Design review of the part built by this model. Coordinates are the model's own, in mm. Face numbers are marked on the shaded views. A direction names the side the tool comes from. Coordinates: 2 decimals unless noted, no trailing zeros. Write each loop counter-clockwise with the first axis right and the second up, starting at its lowest first coordinate (ties: lowest second). Pieces come first, ordered by that corner, then holes. Notation, with made-up numbers: M 29.25,-7 L 43.25,-7 A27 cw 43.25,23 Z; hole C -27.75,33.25 d8. An arc over 180 degrees is marked long. One line per question, with ' | ' between items.
from build123d import *

# Parameters (mm, degrees)
BOSS_EXTRUDE1_DEPTH = 37
SKETCH2_R           = 2
CUT_EXTRUDE1_DEPTH  = 73.566185092
SKETCH3_W           = 30
SKETCH3_H           = 7.896551268
BOSS_EXTRUDE2_DEPTH = 48
SKETCH4_W           = 30
SKETCH4_H           = 6
CUT_EXTRUDE2_DEPTH  = 4
FILLET1_R           = 10
SKETCH5_R           = 5
CUT_EXTRUDE3_DEPTH  = 76.725712885
BOSS_EXTRUDE3_DEPTH = 1
CUT_EXTRUDE4_DEPTH  = 0.5


with BuildPart() as part:
    # Sketch1 → Boss-Extrude1 (new body)
    with BuildSketch(Plane(origin=(0, 0, 0), x_dir=(1, 0, 0), z_dir=(0, 1, 0))):
        with BuildLine():
            Line((0, 0), (6.55816832, -13.490382807))
            ThreePointArc((6.55816832, -13.490382807), (30.474828919, -7.985034321), (54.391489518, -13.490382807))
            Line((54.391489518, -13.490382807), (60.949657838, 0))
            ThreePointArc((60.949657838, 0), (30.474828919, 7.014965679), (0, 0))
        make_face()
    extrude(amount=BOSS_EXTRUDE1_DEPTH)

    # Sketch2 → Cut-Extrude1 (cut, through all)
    with BuildSketch(Plane(origin=(0, 37, 0), x_dir=(1, 0, 0), z_dir=(0, 1, 0))):
        with Locations(Location((12.985948873, -2.622359081, 0), (0, 0, 270))):
            Circle(SKETCH2_R)
        with Locations(Location((47.963708964, -2.622359081, 0), (0, 0, 90))):
            Circle(SKETCH2_R)
    extrude(amount=-CUT_EXTRUDE1_DEPTH, mode=Mode.SUBTRACT)

    # Sketch3 → Boss-Extrude2 (add)
    with BuildSketch(Plane(origin=(0, 37, 0), x_dir=(1, 0, 0), z_dir=(0, 1, 0))):
        with Locations((30.474828919, 8.066690045)):
            Rectangle(SKETCH3_W, SKETCH3_H)
    extrude(amount=-BOSS_EXTRUDE2_DEPTH)

    # Sketch4 → Cut-Extrude2 (cut)
    with BuildSketch(Plane.XY.offset(-4.118414411)):
        with Locations((30.474828919, -3)):
            Rectangle(SKETCH4_W, SKETCH4_H)
    extrude(amount=-CUT_EXTRUDE2_DEPTH, mode=Mode.SUBTRACT)

    # Fillet1
    fillet1_edges = [part.edges().sort_by_distance(p)[0] for p in [
        (15.474828919, -11, -8.066690045),
        (45.474828919, -11, -8.066690045),
    ]]
    fillet(fillet1_edges, radius=FILLET1_R)

    # Sketch5 → Cut-Extrude3 (cut, through all)
    with BuildSketch(Plane(origin=(0, 0, -12.014965679), x_dir=(-1, 0, 0), z_dir=(0, 0, -1))):
        with Locations((-30.474828919, 27)):
            Circle(SKETCH5_R)
    extrude(amount=-CUT_EXTRUDE3_DEPTH, mode=Mode.SUBTRACT)

    # Sketch7 → Boss-Extrude3 (add)
    with BuildSketch(Plane(origin=(0, 0, -12.014965679), x_dir=(-1, 0, 0), z_dir=(0, 0, -1))):
        with BuildLine():
            Line((-21.536068007, 1.453872129), (-26.199769352, 0))
            ThreePointArc((-26.199769352, 0), (-24.751375622, 3.560871216), (-21.536068007, 1.453872129))
        make_face()
        with BuildLine():
            Line((-34.426020337, 3.673663851), (-38.960174422, 5.664158065))
            ThreePointArc((-38.960174422, 5.664158065), (-37.895872331, 1.929105477), (-34.426020337, 3.673663851))
        make_face()
    extrude(amount=BOSS_EXTRUDE3_DEPTH)

    # Sketch8 → Cut-Extrude4 (cut)
    with BuildSketch(Plane(origin=(0, 0, -13.014965679), x_dir=(-1, 0, 0), z_dir=(0, 0, -1))):
        with BuildLine():
            Line((-23.022731531, 0.990416495), (-25.036897729, 0.362516061))
            ThreePointArc((-25.036897729, 0.362516061), (-24.475304572, 2.105499822), (-23.022731531, 0.990416495))
        make_face()
        with BuildLine():
            Line((-35.750767501, 4.255228023), (-37.89390211, 5.196064386))
            ThreePointArc((-37.89390211, 5.196064386), (-37.451768412, 3.29185708), (-35.750767501, 4.255228023))
        make_face()
    extrude(amount=-CUT_EXTRUDE4_DEPTH, mode=Mode.SUBTRACT)


solid = part.part
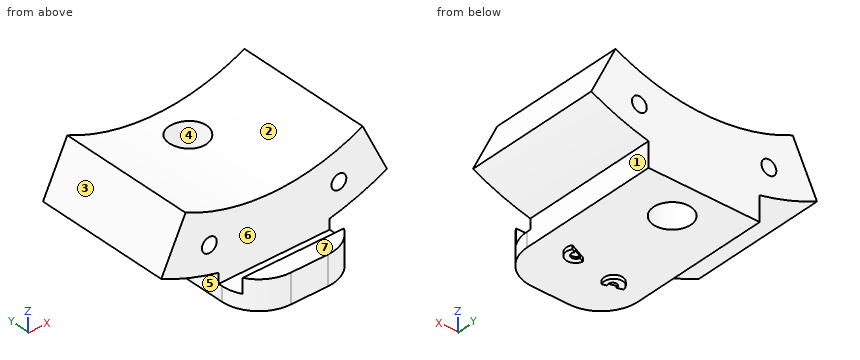
1. Take a section at B-B (y = 31). Write out the cut boundary in (x, z), then the cut area to 3 significant figures.
Answer sheet:
outline: M 0,0 A69.7 ccw 15.47,-5.38 L 15.47,-12.01 L 27.47,-12.01 L 27.47,8.07 A54.7 cw 6.56,13.49 Z; M 33.47,-12.01 L 45.47,-12.01 L 45.47,-5.38 A69.7 ccw 60.95,0 L 54.39,13.49 A54.7 cw 33.47,8.07 Z; hole C 12.99,2.62 d4; hole C 47.96,2.62 d4 | area: 865 mm^2
2. Insertion check: pin 1 Ø1.5 at (x, y) = (35.5, -9) entering from +Z; pin 2 Ø2 at (x, z) = (13.5, 6.5) entering from -Y; pin 3 Ø5 at (x, y) = (31.5, -2) entering from +Z; pin 4 Ø9 at (x, y) = (25.5, 5) entering from -Z. Each pin has a flat end and moves straight along its axis. Give the tip position at first contact, or say it passes through.
Answer sheet:
pin 1: z = -4.12 | pin 2: y = 0 | pin 3: z = 8.04 | pin 4: z = -13.01
3. Draft analysis for pull direction X (two halves, no side actions). For the marked faces 1, 2, 3 and 4, state which applies: pulls with the +X half, pulls with the -X half, needs draft (parallel to the pull), parting line crosses it, or undercut.
Answer sheet:
face 1: pulls with the +X half | face 2: undercut | face 3: pulls with the -X half | face 4: undercut
4. Take a section at A-A (z = -7). Write out the cut boundary in (x, y).
Answer sheet:
outline: M 15.47,0 L 45.47,0 L 45.47,37 L 15.47,37 Z; M 16.81,-6 A10 ccw 25.47,-11 L 35.47,-11 A10 ccw 44.14,-6 Z; hole C 30.47,27 d10
5. Take a section at D-D (z = 5.75). Write out the cut boundary in (x, y), then the cut area to 3 significant figures.
Answer sheet:
outline: M 2.8,0 L 58.15,0 L 58.15,37 L 2.8,37 Z; hole C 30.47,27 d10 | area: 1,970 mm^2
6. Tool access review of the marked faces 5, 6 and 7: name each direction out of +Z, -Z, +X, -X, +Y, -Y from which nothing blocks a thin tool from reaching the whole face with its end or side.
Answer sheet:
face 5: -Z, -X, +Y, -Y | face 6: +Z, +X, -X | face 7: +Z, +X, -X, -Y
7. Take a section at C-C (x = 32.5). Write out the cut boundary in (y, z), then the cut area to 3 significant figures.
Answer sheet:
outline: M -11,-12.01 L 22.43,-12.01 L 22.43,8.02 L 0,8.02 L 0,-8.12 L -6,-8.12 L -6,-4.12 L -11,-4.12 Z; M 31.57,-12.01 L 37,-12.01 L 37,8.02 L 31.57,8.02 Z | area: 621 mm^2
8. To check wall thickness, follow line 1 along X through (y, z) = (12, 4.25); line 2 along Y through (x, z) = (13, 4.75); line 3 along X through (y, z) = (18, -6.25). State the ranges of each line that lie inside material, in increasing order. Write a range as [from, to].
Answer sheet:
line 1: [2.07, 11.82], [14.15, 46.8], [49.13, 58.88] | line 2: [0, 37] | line 3: [15.47, 45.47]
